Design review of the part built by this model. Coordinates are the model's own, in mm. A direction names the side the tool comes from. Coordinates: 2 decimals unless noted, no trailing zeros. Write each loop counter-clockwise with the first axis right and the second up, starting at its lowest first coordinate (ties: lowest second). Pieces come first, ordered by that corner, then holes. Notation, with made-up numbers: (-7.75, 16.5) - (-3.75, 16.5) arc R32 cw to (-3.75, 52.5) - close; hole circle Ø7 at (70.25, 60). An arc over 180 degrees is marked (long way). Answer as a JSON object with one key per item and string values.
```python
from build123d import *

# Parameters (mm, degrees)
F1_DEPTH = 30


with BuildPart() as f1:
    # F0 (on Front) → F1 (new body)
    with BuildSketch(Plane.XZ):
        Polygon((12, 27), (0, 6.21539), (-12, 27), (-27, 27), (-27, 12), (-6.21539, 0), (-27, -12), (-27, -27), (-12, -27), (0, -6.21539), (12, -27), (27, -27), (27.000002, -12), (6.215392, -1e-06), (27.000001, 12), (27, 27), align=None)
    extrude(amount=F1_DEPTH)


solid = f1.part
```
(1) Take a section at A-A, the plane z = -19. Write out the cut boundary in (x, y), and give its area (3 significant figures).
Solved:
{"outline": "(-27, -30) - (-7.38, -30) - (-7.38, 0) - (-27, 0) - close; (7.38, -30) - (27, -30) - (27, 0) - (7.38, 0) - close", "area": "1,180 mm^2"}
(2) Take a section at D-D, the plane x = 2. Write out the cut boundary in (y, z), and give its area (3 significant figures).
Solved:
{"outline": "(-30, -9.68) - (0, -9.68) - (0, 9.68) - (-30, 9.68) - close", "area": "581 mm^2"}
(3) Tool access review of faces 1 (the face through (-16.75, -14.79, 6.08)), 2 (the face through (6.08, -14.79, 16.75)), 3 (the face through (-6.08, -14.79, -16.75)): name each direction out of +Z, -Z, +X, -X, +Y, -Y from which nothing blocks a thin tool from reaching the whole face with its end or side.
Solved:
{"face 1": "-X, +Y, -Y", "face 2": "+Z, +Y, -Y", "face 3": "-Z, +Y, -Y"}
(4) Take a section at C-C, the plane y = -8.75. Write out the cut boundary in (x, z), and give its area (3 significant figures).
Solved:
{"outline": "(-27, -27) - (-12, -27) - (0, -6.22) - (12, -27) - (27, -27) - (27, -12) - (6.22, 0) - (27, 12) - (27, 27) - (12, 27) - (0, 6.22) - (-12, 27) - (-27, 27) - (-27, 12) - (-6.22, 0) - (-27, -12) - close", "area": "1,920 mm^2"}
(5) Take a section at B-B, the plane x = -10.5. Write out the cut boundary in (y, z).
Solved:
{"outline": "(-30, -24.4) - (0, -24.4) - (0, -2.47) - (-30, -2.47) - close; (-30, 2.47) - (0, 2.47) - (0, 24.4) - (-30, 24.4) - close"}
(6) For pin 1 (8 mm diameter, centred on x = 4, y = -26.5, fed in from +Z), flat-tipped, find the tip position at first contact; note if it passes through.
Solved:
{"pin 1": "stops at z = 20.07"}
(7) The part is to be moulded in two halves that separate along Z. For faces 4 (the face through (-27, -15, -19)), 5 (the face through (5.916, -14.79, -16.462)), 6 (the face through (-19, -15, 27)), 7 (the face through (-16.462, -14.79, -5.916)), say which applies: pulls with the +Z half, pulls with the -Z half, needs draft (parallel to the pull), parting line crosses it, or undercut.
Solved:
{"face 4": "needs draft", "face 5": "pulls with the -Z half", "face 6": "pulls with the +Z half", "face 7": "undercut"}
(8) To check wall thickness, follow line 1 (Z direction, x = -13, y = -26.5); line 2 (X direction, y = -22.75, z = 9); line 3 (X direction, y = -18, z = -24.5). State the ranges of each line that lie inside material, in increasing order. Write a range as from..to.
Solved:
{"line 1": "z = -27..-3.92, 3.92..27", "line 2": "x = -21.8..-1.61, 1.61..21.8", "line 3": "x = -27..-10.56, 10.56..27"}
